The listing builds one solid part. Answer for the finished solid, in the listing's coordinates (mm). Face numbers are marked on the shaded views. A direction names the side the tool comes from. Give positions to 0.01 mm unless a question says otherwise; leave off trailing zeros. Loops run counter-clockwise (first coordinate to the right, second up) from the corner with the lowest first, then second, coordinate; pieces in that order, holes last. Notation, with made-up numbers: (9.5, 11.5) - (17.5, 11.5) arc R28 ccw to (17.5, 30.5) - close; hole circle Ø9 at (51.5, 34). An arc over 180 degrees is marked (long way). Answer in a Markdown table with one row per item. Add a question column.
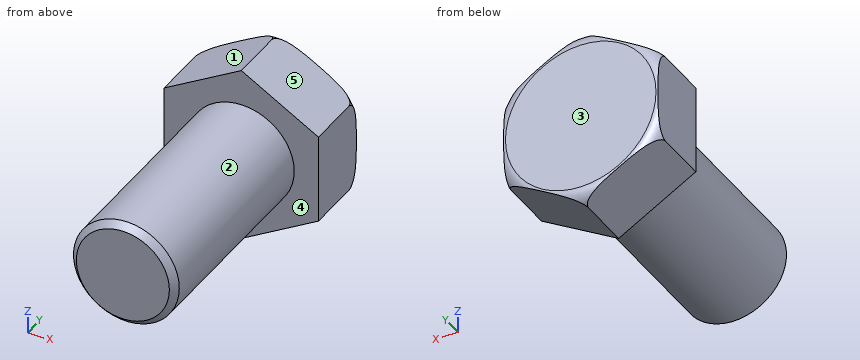
```python
from build123d import *

# Parameters (mm, degrees)
EXTRUDE1_DEPTH = 8.128
SKETCH3_R      = 6.35
EXTRUDE2_DEPTH = 25.4
CHAMFER1_SIZE  = 0.762


with BuildPart() as part:
    # Sketch1 → Extrude1 (new body)
    with BuildSketch(Plane(origin=(0, 0, 0), x_dir=(1, 0, 0), z_dir=(0, 1, 0))):
        Polygon((0, 10.697481421), (-9.264290667, 5.34874071), (-9.264290667, -5.34874071), (0, -10.697481421), (9.264290667, -5.34874071), (9.264290667, 5.34874071), align=None)
    extrude(amount=EXTRUDE1_DEPTH)

    # Sketch3 → Extrude2 (add)
    with BuildSketch(Plane.XZ):
        Circle(SKETCH3_R)
    extrude(amount=EXTRUDE2_DEPTH)

    # Sketch2 → Cut-Revolve1 (revolve, cut)
    with BuildSketch(Plane(origin=(0, 0, 0), x_dir=(0, 0, -1), z_dir=(1, 0, 0))):
        with BuildLine():
            Line((9.038030353, 8.128), (10.697481421, 8.128))
            Line((10.697481421, 8.128), (10.697481421, 6.468548932))
            ThreePointArc((10.697481421, 6.468548932), (10.211439456, 7.641958035), (9.038030353, 8.128))
        make_face()
    revolve(axis=Axis((0, -25.4, 0), (0, 1, 0)), mode=Mode.SUBTRACT)

    # Chamfer1
    chamfer1_edges = [part.edges().sort_by_distance(p)[0] for p in [
        (-6.35, -25.4, 0),
    ]]
    chamfer(chamfer1_edges, length=CHAMFER1_SIZE)


solid = part.part
```
(1) A tool of negligible diameter and unlimited length cuts with its end or side. For the marked faces 4 and 5, from which of +Z, -Z, +X, -X, +Y, -Y can it reach the whole face along a straight path? Write none if from no direction.
(2) A cutting plane is placed at B-B on y = -20.5. Determine the outline of the cut face in (x, z), plus the area to 3 significant figures.
(3) Find the intervals of material crossed by line 1 along Y through (x, z) = (8, 0.5); line 2 along Z through (x, y) = (-3, -19), in increasing order. Write a range as [from, to].
(4) The mould has two halves that part along Z. Classify the marked faces 1, 2 and 3: pulls with the +Z half, pulls with the -Z half, needs draft (parallel to the pull), parting line crosses it, or undercut.
(5) A cutting plane is placed at A-A on z = 0. Determine the outline of the cut face in (x, y).
(6) Given pin 1 Ø2 at (y, z) = (-18, 3.5) entering from +X; pin 2 Ø8 at (x, y) = (-2, 2) entering from -Z; pin 3 Ø6 at (y, z) = (-6.5, 1.5) entering from +X; pin 4 Ø10 at (x, y) = (-1.5, -18) entering from -Z, each flat-ended and moving along its own axis, determine where each tip first touches the part or whether it passes through.
Evaluation:
| question | item | result |
|---|---|---|
| 1 | face 4 | -Y |
| 1 | face 5 | +Z, +X, +Y, -Y |
| 2 | outline | circle Ø12.7 at (0, 0) |
| 2 | area | 127 mm² |
| 3 | line 1 | y = [0, 8.13] |
| 3 | line 2 | z = [-5.6, 5.6] |
| 4 | face 1 | pulls with the +Z half |
| 4 | face 2 | parting line crosses it |
| 4 | face 3 | needs draft |
| 5 | outline | (-9.26, 0) - (-6.35, 0) - (-6.35, -24.64) - (-5.59, -25.4) - (5.59, -25.4) - (6.35, -24.64) - (6.35, 0) - (9.26, 0) - (9.26, 8.11) arc R1.66 ccw to (9.04, 8.13) - (-9.04, 8.13) arc R1.66 ccw to (-9.26, 8.11) - close |
| 6 | pin 1 | stops at x = 5.84 |
| 6 | pin 2 | stops at z = -10.7 |
| 6 | pin 3 | stops at x = 6.35 |
| 6 | pin 4 | stops at z = -6.35 |
